from build123d import *

# Parameters (mm, degrees)
F0_W                 = 30
F0_H                 = 30
F1_DEPTH             = 15
F8_D                 = 6
F8_DEPTH             = 2
F8_CBORE_D           = 6
F8_CBORE_DEPTH       = 2
F8_TIP               = 1.8025818571
F8_ON_F5_D           = 6
F8_ON_F5_DEPTH       = 2
F8_ON_F5_CBORE_D     = 6
F8_ON_F5_CBORE_DEPTH = 2
F8_ON_F5_TIP         = 1.8025818571
F8_ON_F7_D           = 6
F8_ON_F7_DEPTH       = 2
F8_ON_F7_CBORE_D     = 6
F8_ON_F7_CBORE_DEPTH = 2
F8_ON_F7_TIP         = 1.8025818571
F8_ON_F3_D           = 6
F8_ON_F3_DEPTH       = 2
F8_ON_F3_CBORE_D     = 6
F8_ON_F3_CBORE_DEPTH = 2
F8_ON_F3_TIP         = 1.8025818571
F8_ON_F4_D           = 6
F8_ON_F4_DEPTH       = 2
F8_ON_F4_CBORE_D     = 6
F8_ON_F4_CBORE_DEPTH = 2
F8_ON_F4_TIP         = 1.8025818571
F8_ON_F6_D           = 6
F8_ON_F6_DEPTH       = 2
F8_ON_F6_CBORE_D     = 6
F8_ON_F6_CBORE_DEPTH = 2
F8_ON_F6_TIP         = 1.8025818571


with BuildPart() as f1:
    # F0 (on Front) → F1 (new body, symmetric)
    with BuildSketch(Plane.XZ):
        Rectangle(F0_W, F0_H)
    extrude(amount=F1_DEPTH, both=True)

    # F8
    with Locations(Plane.XZ.offset(15)):
        with Locations((7.5, 7.5), (0, 0), (-7.5, -7.5)):
            CounterBoreHole(F8_D / 2, F8_CBORE_D / 2, F8_CBORE_DEPTH, depth=F8_DEPTH)
            with Locations((0, 0, -(F8_DEPTH + F8_TIP / 2))):  # 118° drill point
                Cone(0, F8_D / 2, F8_TIP, mode=Mode.SUBTRACT)

    # F8 on F5
    with Locations(Plane(origin=(0, 15, 0), x_dir=(-1, 0, 0), z_dir=(0, 1, 0))):
        with Locations((-7.5, 7.5), (7.5, 7.5), (7.5, -7.5), (-7.5, -7.5)):
            CounterBoreHole(F8_ON_F5_D / 2, F8_ON_F5_CBORE_D / 2, F8_ON_F5_CBORE_DEPTH, depth=F8_ON_F5_DEPTH)
            with Locations((0, 0, -(F8_ON_F5_DEPTH + F8_ON_F5_TIP / 2))):  # 118° drill point
                Cone(0, F8_ON_F5_D / 2, F8_ON_F5_TIP, mode=Mode.SUBTRACT)

    # F8 on F7
    with Locations(Plane(origin=(-15, 0, 0), x_dir=(0, -1, 0), z_dir=(-1, 0, 0))):
        with Locations((-7.5, 7.5), (-7.5, 0), (-7.5, -7.5), (7.5, -7.5), (7.5, 0), (7.5, 7.5)):
            CounterBoreHole(F8_ON_F7_D / 2, F8_ON_F7_CBORE_D / 2, F8_ON_F7_CBORE_DEPTH, depth=F8_ON_F7_DEPTH)
            with Locations((0, 0, -(F8_ON_F7_DEPTH + F8_ON_F7_TIP / 2))):  # 118° drill point
                Cone(0, F8_ON_F7_D / 2, F8_ON_F7_TIP, mode=Mode.SUBTRACT)

    # F8 on F3
    with Locations(Plane.YZ.offset(15)):
        with Locations((0, 0)):
            CounterBoreHole(F8_ON_F3_D / 2, F8_ON_F3_CBORE_D / 2, F8_ON_F3_CBORE_DEPTH, depth=F8_ON_F3_DEPTH)
            with Locations((0, 0, -(F8_ON_F3_DEPTH + F8_ON_F3_TIP / 2))):  # 118° drill point
                Cone(0, F8_ON_F3_D / 2, F8_ON_F3_TIP, mode=Mode.SUBTRACT)

    # F8 on F4
    with Locations(Plane.XY.offset(15)):
        with Locations((-7.5, 7.5), (7.5, -7.5)):
            CounterBoreHole(F8_ON_F4_D / 2, F8_ON_F4_CBORE_D / 2, F8_ON_F4_CBORE_DEPTH, depth=F8_ON_F4_DEPTH)
            with Locations((0, 0, -(F8_ON_F4_DEPTH + F8_ON_F4_TIP / 2))):  # 118° drill point
                Cone(0, F8_ON_F4_D / 2, F8_ON_F4_TIP, mode=Mode.SUBTRACT)

    # F8 on F6
    with Locations(Plane(origin=(0, 0, -15), x_dir=(1, 0, 0), z_dir=(0, 0, -1))):
        with Locations((-7.5, -7.5), (0, 0), (7.5, 7.5), (-7.5, 7.5), (7.5, -7.5)):
            CounterBoreHole(F8_ON_F6_D / 2, F8_ON_F6_CBORE_D / 2, F8_ON_F6_CBORE_DEPTH, depth=F8_ON_F6_DEPTH)
            with Locations((0, 0, -(F8_ON_F6_DEPTH + F8_ON_F6_TIP / 2))):  # 118° drill point
                Cone(0, F8_ON_F6_D / 2, F8_ON_F6_TIP, mode=Mode.SUBTRACT)


solid = f1.part
Model file for the job. Use its own axes, mm. A direction names the side the tool comes from. Give positions to 0.01 mm unless a question says otherwise; leave off trailing zeros. Order: outer loops, then holes, each group sorted by start corner. A loop starts at its lowest first (then second) coordinate and runs counter-clockwise, first axis right, second up. Notation, with made-up numbers: M 30.5,-11.75 L 44.5,-11.75 A21 cw 44.5,9.25 Z; hole C 33,73.25 d8. An arc over 180 degrees is marked long. Put each result on its own line as item: value. Start each with the question number.
(1) Band-saw the part on A-A on x = 12.5. Give the cut face in (y, z), then the cut area to 3 significant figures.
(2) Pull direction Y, two halves, no side cores. Call faces 1 (the face through (-15, 0, 0)), 2 (the face through (-10.27, -6.35, -13.99)), 3 (the face through (7.8, -11.5, 7.9)): released by +Y, released by -Y, zero draft, split by the parting line, or undercut.
(3) Tool access for faces 4 (the face through (-13.99, -4.64, 8.4)), 5 (the face through (-4.64, 13.99, 8.4)), 6 (the face through (4.64, -8.4, -13.99)): list every direction of +Z, -Z, +X, -X, +Y, -Y with a clear straight run to the whole face (end or side of a thin tool).
(4) Pin check, flat tips, straight feed: pin 1 Ø8 at (x, y) = (-7.5, 7.5) entering from -Z; pin 2 Ø5 at (x, z) = (-7.5, -7.5) entering from -Y; pin 3 Ø5.5 at (x, z) = (7.5, 7.5) entering from +Y; pin 4 Ø5.5 at (x, y) = (7.5, -7.5) entering from +Z. Stop position of each tip, or through.
(5) Drill centre lines: L1, parallel to X at y = 13.5, z = -7.5; L2, parallel to Z at x = -14.6, y = 7.5. Where is each one in solid material? Low to high. Write a range as [from, to].
Results below:
1. outline: M -15,-15 L 15,-15 L 15,15 L -15,15 Z; hole C 0,0 d4.34
1. area: 885 mm2
2. face 1: zero draft
2. face 2: undercut
2. face 3: released by -Y
3. face 4: -X
3. face 5: +Y
3. face 6: -Z
4. pin 1: stops at z = -15
4. pin 2: stops at y = -12.7
4. pin 3: stops at y = 12.85
4. pin 4: stops at z = 12.85
5. L1: x = [-15, -10.5], [-4.5, 4.5], [10.5, 15]
5. L2: z = [-15, -10.5], [-4.5, -3], [3, 4.5], [10.5, 15]
